Geometry: final body of the model. Coordinates: model frame, mm. A direction names the side the tool comes from. Give positions to 0.01 mm unless a question says otherwise; leave off trailing zeros. Write each loop counter-clockwise with the first axis right and the second up, starting at its lowest first coordinate (ties: lowest second). Pieces come first, ordered by that corner, then holes.
Q1. Draft query along Z for faces 4 (the face through (1, 2, -7.95)), 5 (the face through (2.8, 0, -9)), 6 (the face through (0.267, 2.033, -9.218)), 7 (the face through (4, 0, -10.15)). Return one class per face: pulls with the +Z half, pulls with the -Z half, needs draft (parallel to the pull), parting line crosses it, or undercut.
Q2. Pin query (flat end, axial travel): pin 1 (3 mm diameter, centred on x = -3.5, z = -6, fed in from -Y); pin 2 (1.1 mm diameter, centred on y = 0, z = -7, fed in from +X); pin 3 (0.7 mm diameter, centred on y = -0.5, z = -9, fed in from -X). Return the tip coordinate at first contact, or that it passes through.
Q3. Cut plane B-B on x = -0.25. Return the cut outline in (y, z) (3 decimals), plus the area to 3 significant figures.
Q4. Reachability of faces 1 (the face through (-2, -1, -10.45)), 2 (the face through (5.492, 0, -7)), 3 (the face through (-2.8, 0, -9)) from +Z, -Z, +X, -X, +Y, -Y: full face, straight path, thin tool, end or side. Return the list, or none.
Q5. Cut plane C-C on y = -2.75. Count the separate pieces of the cut face and the enclosed holes in it, plus the area to 3 significant figures.
Q6. Line query: L1, parallel to Y at x = 0, z = -10.5; L2, parallel to Y at x = 0, z = -9.6; L3, parallel to X at y = 0.5, z = -7. Output: solid intervals per line, ascending.
```python
from build123d import *

# Parameters (mm, degrees)
BOSS_EXTRUDE1_DEPTH = 6.5
SKETCH5_R           = 2.05
CUT_EXTRUDE2_DEPTH  = 12.301797423
SKETCH6_R           = 3.05
CUT_EXTRUDE3_DEPTH  = 0.2
FILLET1_R           = 6.5
SKETCH7_W           = 6.3
SKETCH7_H           = 6.3
CUT_EXTRUDE4_DEPTH  = 3.875


with BuildPart() as part:
    # Sketch2 → Boss-Extrude1 (new, symmetric)
    with BuildSketch(Plane(origin=(0, 0, 0), x_dir=(1, 0, 0), z_dir=(0, 1, 0))):
        with BuildLine():
            Line((-2.8, 10), (-2.8, 10.15))
            Line((-2.8, 10.15), (-6.5, 10.15))
            Line((-6.5, 10.15), (-6.5, 10.65))
            Line((-6.5, 10.65), (6.5, 10.65))
            Line((6.5, 10.65), (6.5, 10.15))
            Line((6.5, 10.15), (2.8, 10.15))
            Line((2.8, 10.15), (2.8, 10))
            Line((2.8, 10), (2.8, 7.9))
            Line((2.8, 7.9), (5.492157288, 7.9))
            Line((5.492157288, 7.9), (5.492157288, 6.65))
            Line((5.492157288, 6.65), (3.151471863, 4.309314575))
            ThreePointArc((3.151471863, 4.309314575), (2.891933184, 4.135896374), (2.585786438, 4.075))
            Line((2.585786438, 4.075), (-2.585786438, 4.075))
            ThreePointArc((-2.585786438, 4.075), (-2.891933184, 4.135896374), (-3.151471863, 4.309314575))
            Line((-3.151471863, 4.309314575), (-5.492157288, 6.65))
            Line((-5.492157288, 6.65), (-5.492157288, 7.9))
            Line((-5.492157288, 7.9), (-2.8, 7.9))
            Line((-2.8, 7.9), (-2.8, 10))
        make_face()
    extrude(amount=BOSS_EXTRUDE1_DEPTH, both=True)

    # Sketch5 → Cut-Extrude2 (cut, through all)
    with BuildSketch(Plane(origin=(0, 0, -10.65), x_dir=(-1, 0, 0), z_dir=(0, 0, -1))):
        Circle(SKETCH5_R)
    extrude(amount=-CUT_EXTRUDE2_DEPTH, mode=Mode.SUBTRACT)

    # Sketch6 → Cut-Extrude3 (cut)
    with BuildSketch(Plane(origin=(0, 0, -10.65), x_dir=(-1, 0, 0), z_dir=(0, 0, -1))):
        Circle(SKETCH6_R)
    extrude(amount=-CUT_EXTRUDE3_DEPTH, mode=Mode.SUBTRACT)

    # Fillet1
    fillet1_edges = [part.edges().sort_by_distance(p)[0] for p in [
        (6.5, -6.5, -10.4),
        (-6.5, -6.5, -10.4),
        (6.5, 6.5, -10.4),
        (-6.5, 6.5, -10.4),
    ]]
    fillet(fillet1_edges, radius=FILLET1_R - 0.0001)  # a hair under: the kernel refuses the full size

    # Sketch7 → Cut-Extrude4 (cut)
    with BuildSketch(Plane.XY.offset(-4.075)):
        Rectangle(SKETCH7_W, SKETCH7_H)
    extrude(amount=-CUT_EXTRUDE4_DEPTH, mode=Mode.SUBTRACT)


solid = part.part
```
Data:
1. face 4: pulls with the +Z half
1. face 5: undercut
1. face 6: needs draft
1. face 7: undercut
2. pin 1: stops at y = -6.18
2. pin 2: stops at x = 5.49
2. pin 3: stops at x = -2.8
3. outline: (-6.495, -10.65) - (-3.04, -10.65) - (-3.04, -10.45) - (-2.035, -10.45) - (-2.035, -7.95) - (-3.15, -7.95) - (-3.15, -4.075) - (-6.495, -4.075) - close; (2.035, -10.45) - (3.04, -10.45) - (3.04, -10.65) - (6.495, -10.65) - (6.495, -4.075) - (3.15, -4.075) - (3.15, -7.95) - (2.035, -7.95) - close
3. area: 49.6 mm2
4. face 1: -Z
4. face 2: +Z, +X, +Y, -Y
4. face 3: -X, +Y, -Y
5. separate pieces: 3
5. enclosed holes: 0
5. area: 29.0 mm2
6. L1: y = -6.5 to -3.05, 3.05 to 6.5
6. L2: y = -6.5 to -2.05, 2.05 to 6.5
6. L3: x = -5.49 to -3.15, 3.15 to 5.49
